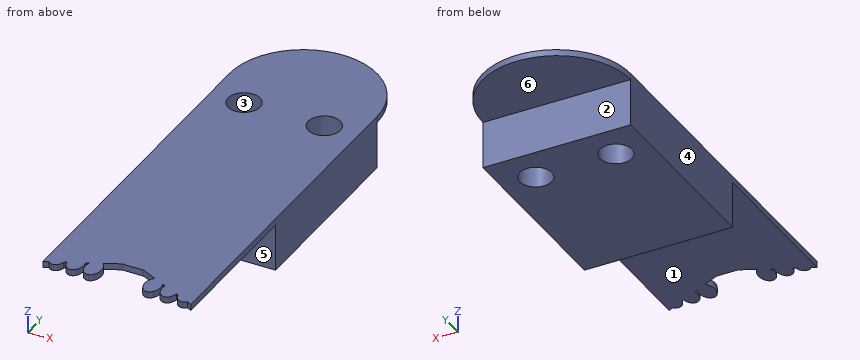
```python
from build123d import *

# Parameters (mm, degrees)
SKETCH1_W           = 46.787939469
SKETCH1_H           = 60
SKETCH1_R           = 5.08
BOSS_EXTRUDE1_DEPTH = 15
SKETCH2_W           = 46.787939469
SKETCH2_H           = 60
SKETCH2_R           = 5.08
BOSS_EXTRUDE2_DEPTH = 2


with BuildPart() as part:
    # Sketch1 → Boss-Extrude1 (new body)
    with BuildSketch(Plane.XY):
        with Locations((-102.767623853, -313.368909969)):
            Rectangle(SKETCH1_W, SKETCH1_H)
        with Locations((-90.073654119, -294.630909969)):
            Circle(SKETCH1_R, mode=Mode.SUBTRACT)
        with Locations((-115.461593588, -294.630909969)):
            Circle(SKETCH1_R, mode=Mode.SUBTRACT)
    extrude(amount=BOSS_EXTRUDE1_DEPTH)

    # Sketch2 → Boss-Extrude2 (add)
    with BuildSketch(Plane.XY.offset(15)):
        with BuildLine():
            Line((-79.373654119, -343.368909969), (-102.767623854, -343.368909969))
            Line((-102.767623854, -343.368909969), (-102.767623854, -384.042756806))
            Line((-102.767623854, -384.042756806), (-99.373654119, -384.042756806))
            Line((-99.373654119, -384.042756806), (-94.503579918, -386.313709702))
            add(Edge.make_bspline(
                [(-94.503579918, -386.313709702), (-100.00398624, -390.494082743), (-94.115799531, -393.239789298), (-93.929989905, -393.32643375), (-93.73748043, -393.368909969)],
                knots=[0.468972903, 0.468972903, 0.468972903, 2.84019184, 2.84019184, 3.029420352, 3.029420352, 3.029420352], degree=2, weights=[1, 0.37573231, 1, 0.950182059, 0.908315281]))
            Line((-93.73748043, -393.368909969), (-93.009827808, -393.368909969))
            add(Edge.make_bspline(
                [(-93.009827808, -393.368909969), (-89.462741956, -392.586263836), (-91.178526324, -387.864207656)],
                knots=[3.345008297, 3.345008297, 3.345008297, 5.211410777, 5.211410777, 5.211410777], degree=2, weights=[0.790783298, 0.508634675, 1]))
            Line((-91.178526324, -387.864207656), (-90.208062599, -388.316742323))
            add(Edge.make_bspline(
                [(-90.208062599, -388.316742323), (-91.162547167, -392.052221372), (-88.615799531, -393.239789298), (-88.429989905, -393.32643375), (-88.23748043, -393.368909969)],
                knots=[1.204788076, 1.204788076, 1.204788076, 2.84019184, 2.84019184, 3.008967996, 3.008967996, 3.008967996], degree=2, weights=[1, 0.683899664, 1, 0.967377965, 0.941489216]))
            Line((-88.23748043, -393.368909969), (-87.509827808, -393.368909969))
            add(Edge.make_bspline(
                [(-87.509827808, -393.368909969), (-85.839475159, -393.000355303), (-85.443416113, -390.538533468)],
                knots=[3.304458938, 3.304458938, 3.304458938, 4.475595603, 4.475595603, 4.475595603], degree=2, weights=[0.871477119, 0.773635905, 1]))
            Line((-85.443416113, -390.538533468), (-84.740509949, -390.866303995))
            add(Edge.make_bspline(
                [(-84.740509949, -390.866303995), (-84.248679529, -393.03547171), (-82.73748043, -393.368909969)],
                knots=[1.898629299, 1.898629299, 1.898629299, 2.984182814, 2.984182814, 2.984182814], degree=2, weights=[1, 0.762799808, 0.799074283]))
            Line((-82.73748043, -393.368909969), (-82.009827808, -393.368909969))
            add(Edge.make_bspline(
                [(-82.009827808, -393.368909969), (-81.386018968, -393.231269777), (-80.880341234, -392.666330229)],
                knots=[3.261132643, 3.261132643, 3.261132643, 3.781754381, 3.781754381, 3.781754381], degree=2, weights=[0.83538307, 0.886240914, 1]))
            Line((-80.880341234, -392.666330229), (-79.373654119, -393.368909969))
            Line((-79.373654119, -393.368909969), (-79.373654119, -343.368909969))
        make_face()
        with BuildLine():
            Line((-126.161593588, -343.368909969), (-126.161593588, -393.368909969))
            Line((-126.161593588, -393.368909969), (-124.654906474, -392.666330229))
            add(Edge.make_bspline(
                [(-124.654906474, -392.666330229), (-124.14922874, -393.231269777), (-123.525419899, -393.368909969)],
                knots=[2.501430927, 2.501430927, 2.501430927, 3.022052664, 3.022052664, 3.022052664], degree=2, weights=[1, 0.886240914, 0.83538307]))
            Line((-123.525419899, -393.368909969), (-122.797767278, -393.368909969))
            add(Edge.make_bspline(
                [(-122.797767278, -393.368909969), (-121.286568178, -393.03547171), (-120.794737759, -390.866303995)],
                knots=[3.299002493, 3.299002493, 3.299002493, 4.384556008, 4.384556008, 4.384556008], degree=2, weights=[0.799074283, 0.762799808, 1]))
            Line((-120.794737759, -390.866303995), (-120.091831594, -390.538533468))
            add(Edge.make_bspline(
                [(-120.091831594, -390.538533468), (-119.695772548, -393.000355303), (-118.025419899, -393.368909969)],
                knots=[1.807589704, 1.807589704, 1.807589704, 2.97872637, 2.97872637, 2.97872637], degree=2, weights=[1, 0.773635905, 0.871477119]))
            Line((-118.025419899, -393.368909969), (-117.297767278, -393.368909969))
            add(Edge.make_bspline(
                [(-117.297767278, -393.368909969), (-117.105257803, -393.32643375), (-116.919448176, -393.239789298), (-114.37270054, -392.052221372), (-115.327185108, -388.316742323)],
                knots=[3.274217312, 3.274217312, 3.274217312, 3.442993467, 3.442993467, 5.078397231, 5.078397231, 5.078397231], degree=2, weights=[0.941489216, 0.967377965, 1, 0.683899664, 1]))
            Line((-115.327185108, -388.316742323), (-114.356721383, -387.864207656))
            add(Edge.make_bspline(
                [(-114.356721383, -387.864207656), (-116.072505751, -392.586263836), (-112.525419899, -393.368909969)],
                knots=[1.071774531, 1.071774531, 1.071774531, 2.93817701, 2.93817701, 2.93817701], degree=2, weights=[1, 0.508634675, 0.790783298]))
            Line((-112.525419899, -393.368909969), (-111.797767278, -393.368909969))
            add(Edge.make_bspline(
                [(-111.797767278, -393.368909969), (-111.605257803, -393.32643375), (-111.419448176, -393.239789298), (-105.531261468, -390.494082743), (-111.031667789, -386.313709702)],
                knots=[3.253764955, 3.253764955, 3.253764955, 3.442993467, 3.442993467, 5.814212404, 5.814212404, 5.814212404], degree=2, weights=[0.908315281, 0.950182059, 1, 0.37573231, 1]))
            Line((-111.031667789, -386.313709702), (-106.161593588, -384.042756806))
            Line((-106.161593588, -384.042756806), (-102.767623854, -384.042756806))
            Line((-102.767623854, -384.042756806), (-102.767623854, -343.368909969))
            Line((-102.767623854, -343.368909969), (-126.161593588, -343.368909969))
        make_face()
        with Locations((-102.767623853, -313.368909969)):
            Rectangle(SKETCH2_W, SKETCH2_H)
        with Locations((-115.461593588, -294.630909969)):
            Circle(SKETCH2_R, mode=Mode.SUBTRACT)
        with Locations((-90.073654119, -294.630909969)):
            Circle(SKETCH2_R, mode=Mode.SUBTRACT)
        with BuildLine():
            ThreePointArc((-79.373654119, -283.368909969), (-102.767623854, -259.974940234), (-126.161593588, -283.368909969))
            Line((-126.161593588, -283.368909969), (-79.373654119, -283.368909969))
        make_face()
    extrude(amount=BOSS_EXTRUDE2_DEPTH)


solid = part.part
```
For this review, take the finished solid that the model builds, in its own axes (mm). Face numbers are marked on the shaded views. A direction names the side the tool comes from. Coordinates: 2 decimals unless noted, no trailing zeros. Loops run counter-clockwise (first coordinate to the right, second up) from the corner with the lowest first, then second, coordinate; pieces in that order, holes last. Notation, with made-up numbers: (33, 23.5) - (57, 23.5) arc R14 cw to (57, 35.5) - close; hole circle Ø7 at (25.25, -10). An arc over 180 degrees is marked (long way). Use one line per item in the form item = value. Start each with the question number.
1) Take a section at D-D (y = -268). State the section outline as (x, z) points, plus the area to 3 significant figures.
2) Take a section at C-C (y = -357). State the section outline as (x, z) points.
3) For pin 1 (0.6 mm diameter, centred on x = -102, z = 15.5, fed in from -Y); pin 2 (3 mm diameter, centred on x = -109.5, y = -300.5, fed in from -Z); pin 3 (10 mm diameter, centred on x = -96, y = -374.5, fed in from -Z); pin 4 (9 mm diameter, centred on x = -115.46, y = -294.63, fed in from -Z), all flat-tipped, find the tip position at first contact; note any pin that passes through.
4) Take a section at B-B (x = -102.5). State the section outline as (y, z) points, plus the area to 3 significant figures.
5) Draft analysis for pull direction Y (two halves, no side actions). For the marked faces 1, 2 and 3, state which applies: released by +Y, released by -Y, zero draft, split by the parting line, or undercut.
6) For the marked faces 4, 5 and 6, list the 3-axis set-ups (+Z, -Z, +X, -X, +Y, -Y) from which the entire face can be reached by the end or side of a thin tool; tool diameter is ignored.
7) Take a section at A-A (z = 4). State the section outline as (x, y) points.
8) To check wall thickness, follow probe 1 along Y at (x, z) = (-116, 6.75); probe 2 along Y at (x, z) = (-121, 12.25); probe 3 along Y at (x, z) = (-88.5, 11.5). State the ranges of each line that lie inside material, in increasing order. Write a range as from..to.
From the geometry:
q1.outline = (-120.4, 15) - (-85.13, 15) - (-85.13, 17) - (-120.4, 17) - close
q1.area = 70.5 mm2
q2.outline = (-126.16, 15) - (-79.37, 15) - (-79.37, 17) - (-126.16, 17) - close
q3.pin_1 = -384.04
q3.pin_2 = 0
q3.pin_3 = 15
q3.pin_4 = through
q4.outline = (-384.04, 15) - (-343.37, 15) - (-343.37, 0) - (-283.37, 0) - (-283.37, 15) - (-259.98, 15) - (-259.98, 17) - (-384.04, 17) - close
q4.area = 1,150 mm2
q5.face_1 = zero draft
q5.face_2 = released by +Y
q5.face_3 = undercut
q6.face_4 = +Z, -Z, -X, +Y, -Y
q6.face_5 = -Z, +X, -X, -Y
q6.face_6 = -Z, +X, -X, +Y
q7.outline = (-126.16, -343.37) - (-79.37, -343.37) - (-79.37, -283.37) - (-126.16, -283.37) - close; hole circle Ø10.16 at (-115.46, -294.63); hole circle Ø10.16 at (-90.07, -294.63)
q8.probe_1 = -343.37..-299.68, -289.58..-283.37
q8.probe_2 = -343.37..-283.37
q8.probe_3 = -343.37..-299.46, -289.8..-283.37
